Geometry check sheet. Reference: the model listing, model coordinates, mm. A direction names the side the tool comes from. Round coordinates to 2 decimals unless told otherwise and drop trailing zeros. Write each loop counter-clockwise with the first axis right and the second up, starting at its lowest first coordinate (ties: lowest second). Pieces come first, ordered by that corner, then holes.
Item 1: Scan lines: probe 1 along X at (y, z) = (4.25, -10); probe 2 along X at (y, z) = (5, 0); probe 3 along X at (y, z) = (4.75, -2.5). Record each from-to range of solid material in increasing order.
Item 2: Cross-section at D-D (x = 25). Enter the section's corners in (y, z), then the cut area to 3 significant figures.
Item 3: Cross-section at B-B (z = 0). Enter the section's corners in (x, y).
Item 4: Draft check along X on faces 1 (the face through (0, 0, -7)), 2 (the face through (25.537, 3.451, -0.202)), 3 (the face through (29, 3, -2)). Enter one of: pulls with the +X half, pulls with the -X half, needs draft (parallel to the pull), parting line crosses it, or undercut.
Item 5: Access from +Z, -Z, +X, -X, +Y, -Y to the whole of each face (thin tool, end or side, straight path). Record for faces 4 (the face through (27, 4, -14)), 5 (the face through (0, 2, -5)), 6 (the face through (-19.57, 6.4, 0.1)).
Item 6: Cross-section at A-A (z = 3). Enter the section's corners in (x, y).
Item 7: Depth check by flat-ended pin: P1, Ø2.5, axis at x = 0.5, y = 3, coming from the +Z side. Enter the tip coordinate at first touch or a pass-through.
Item 8: Cross-section at C-C (y = 4.5). Enter the section's corners in (x, z).
from build123d import *

# Parameters (mm, degrees)
CROQUIS1_R              = 1.55
SALIENTE_EXTRUIR1_DEPTH = 7
REDONDEO2_R             = 2
REDONDEO3_R             = 5


with BuildPart() as part:
    # Croquis1 → Saliente-Extruir1 (new body)
    with BuildSketch(Plane(origin=(0, 0, 0), x_dir=(1, 0, 0), z_dir=(0, 1, 0))):
        Polygon((-29, -7), (-29, 15), (29, 15), (29, -7), (19, -7), (19, 5), (-19, 5), (-19, -7), align=None)
        with Locations(Location((-24, 0, 0), (0, 0, 270))):
            Circle(CROQUIS1_R, mode=Mode.SUBTRACT)
        with Locations(Location((24, 0, 0), (0, 0, 270))):
            Circle(CROQUIS1_R, mode=Mode.SUBTRACT)
        with Locations(Location((-24, 10, 0), (0, 0, 270))):
            Circle(CROQUIS1_R, mode=Mode.SUBTRACT)
        with Locations(Location((24, 10, 0), (0, 0, 270))):
            Circle(CROQUIS1_R, mode=Mode.SUBTRACT)
    extrude(amount=SALIENTE_EXTRUIR1_DEPTH)

    # Redondeo2
    redondeo2_edges = [part.edges().sort_by_distance(p)[0] for p in [
        (0, 7, -5),
        (19, 7, 1),
        (-19, 7, 1),
    ]]
    fillet(redondeo2_edges, radius=REDONDEO2_R)

    # Redondeo3
    redondeo3_edges = [part.edges().sort_by_distance(p)[0] for p in [
        (-29, 3.5, -15),
        (29, 3.5, -15),
    ]]
    fillet(redondeo3_edges, radius=REDONDEO3_R)


solid = part.part
Resolved:
1. probe 1: x = -29 to -25.55, -22.45 to 22.45, 25.55 to 29
1. probe 2: x = -29 to -25.55, -22.45 to -19, 19 to 22.45, 25.55 to 29
1. probe 3: x = -29 to -19, 19 to 29
2. outline: (0, -14.9) - (7, -14.9) - (7, -11.18) - (0, -11.18) - close; (0, -8.82) - (7, -8.82) - (7, -1.18) - (0, -1.18) - close; (0, 1.18) - (7, 1.18) - (7, 7) - (0, 7) - close
2. area: 120 mm2
3. outline: (-29, 0) - (-25.55, 0) - (-25.55, 7) - (-29, 7) - close; (-22.45, 0) - (-19, 0) - (-19, 5) arc R2 ccw to (-21, 7) - (-22.45, 7) - close; (19, 0) - (22.45, 0) - (22.45, 7) - (21, 7) arc R2 ccw to (19, 5) - close; (25.55, 0) - (29, 0) - (29, 7) - (25.55, 7) - close
4. face 1: needs draft
4. face 2: undercut
4. face 3: pulls with the +X half
5. face 4: -Z, +X, +Y, -Y
5. face 5: +Z, +Y, -Y
5. face 6: +Z, +Y
6. outline: (-29, 0) - (-19, 0) - (-19, 5) arc R2 ccw to (-21, 7) - (-29, 7) - close; (19, 0) - (29, 0) - (29, 7) - (21, 7) arc R2 ccw to (19, 5) - close
7. P1: stops at z = -5
8. outline: (-29, -10) arc R5 ccw to (-24, -15) - (24, -15) arc R5 ccw to (29, -10) - (29, 7) - (19, 7) - (19, -5) - (-19, -5) - (-19, 7) - (-29, 7) - close; hole circle Ø3.1 at (-24, -10); hole circle Ø3.1 at (-24, 0); hole circle Ø3.1 at (24, -10); hole circle Ø3.1 at (24, 0)
